```python
from build123d import *

# Parameters (mm, degrees)
CIRPATTERN1_COUNT              = 8
F_1_4_0_2500_DOWEL_HOLE1_D     = 6.35
F_1_4_0_2500_DOWEL_HOLE1_DEPTH = 9.906
F_1_4_0_2500_DOWEL_HOLE1_TIP   = 1.907732465


with BuildPart() as part:
    # Sketch1 → Revolve2 (revolve)
    with BuildSketch(Plane.XY, mode=Mode.PRIVATE) as revolve2_sk:
        with BuildLine():
            Line((71.727523602, 109.927507641), (76.194467874, 109.927507641))
            Line((76.194467874, 109.927507641), (76.194467874, -212.127513222))
            Line((76.194467874, -212.127513222), (53.881527661, -212.127513222))
            Line((53.881527661, -212.127513222), (53.881527661, -59.727513222))
            add(Edge.make_bspline(
                [(53.881527661, -59.727513222), (53.88152643, -59.656983156), (53.880997287, -59.515406102), (53.878621437, -59.181564616), (53.872296838, -58.904795492), (53.862811351, -58.532567487), (53.850168453, -58.212837621), (53.830417626, -57.781594442), (53.800405285, -57.280959899), (53.756193121, -56.687998165), (53.677288452, -55.848480365), (53.577426861, -55.00816586), (53.456675786, -54.17243543), (53.286810822, -53.172425239), (53.092064187, -52.177442821), (52.86637512, -51.188539083), (52.610014224, -50.207489038), (52.32928934, -49.23307774), (52.024348739, -48.265969223), (51.633537831, -47.149135067), (51.139520361, -45.890408405), (50.598733752, -44.650968803), (50.012060927, -43.432701525), (49.38012023, -42.237093238), (48.704125229, -41.066154878), (47.984475519, -39.920972657), (47.223102138, -38.804076239), (46.51986906, -37.851451785), (45.893537937, -37.055672122), (45.35281768, -36.403381282), (44.915126948, -35.894247632), (44.514776189, -35.446992657), (44.181457503, -35.084631185), (43.873924624, -34.760340151), (43.674072406, -34.55154945), (43.444392072, -34.318516287), (43.343783151, -34.217162055), (43.293911001, -34.167289665)],
                knots=[0.082637729, 0.082637729, 0.082637729, 0.082637729, 0.082637729, 0.092574926, 0.102512123, 0.11244932, 0.122386517, 0.132323714, 0.142260911, 0.162135305, 0.182009699, 0.201884093, 0.24163288, 0.261507274, 0.281381668, 0.321130456, 0.360879243, 0.380753637, 0.400628031, 0.440376819, 0.480125606, 0.519874394, 0.559623181, 0.599371969, 0.639120757, 0.678869544, 0.718618332, 0.75836712, 0.798115907, 0.817990301, 0.837864695, 0.857739089, 0.877613483, 0.88755068, 0.897487877, 0.907425074, 0.91736227, 0.91736227, 0.91736227, 0.91736227, 0.91736227], degree=4))
            Line((43.293911001, -34.167289665), (34.686282803, -25.559661468))
            add(Edge.make_bspline(
                [(24.099067874, 0.000160672), (24.099069105, -0.070367974), (24.099598252, -0.213423517), (24.101973937, -0.543022243), (24.108298331, -0.823999723), (24.117783452, -1.194661398), (24.130425744, -1.513274385), (24.146225968, -1.86177893), (24.165181227, -2.193546199), (24.192818841, -2.617908727), (24.232287047, -3.121873274), (24.303299707, -3.879818002), (24.423126678, -4.886289716), (24.599486044, -6.056550088), (24.850885233, -7.385005743), (25.151795313, -8.703413844), (25.501770623, -10.009476539), (25.900360983, -11.301658928), (26.346945392, -12.577938667), (26.841003323, -13.836726817), (27.381673122, -15.076036463), (27.968479387, -16.294449129), (28.600139398, -17.489778131), (29.276532396, -18.661127096), (29.995445102, -19.805582737), (30.758021999, -20.923699417), (31.459167193, -21.874251104), (32.088736123, -22.673284825), (32.624128416, -23.320261484), (33.072255768, -23.839844364), (33.508450026, -24.329655594), (33.935826121, -24.788323739), (34.24555864, -25.11370766), (34.536859958, -25.409488397), (34.636412426, -25.509789283), (34.686282803, -25.559661468)],
                knots=[0.082637729, 0.082637729, 0.082637729, 0.082637729, 0.082637729, 0.092574926, 0.102512123, 0.11244932, 0.122386517, 0.132323714, 0.142260911, 0.152198108, 0.162135305, 0.182009699, 0.201884093, 0.24163288, 0.281381668, 0.321130456, 0.360879243, 0.400628031, 0.440376819, 0.480125606, 0.519874394, 0.559623181, 0.599371969, 0.639120757, 0.678869544, 0.718618332, 0.75836712, 0.798115907, 0.817990301, 0.837864695, 0.857739089, 0.877613483, 0.897487877, 0.907425074, 0.91736227, 0.91736227, 0.91736227, 0.91736227, 0.91736227], degree=4))
            add(Edge.make_bspline(
                [(24.099067874, 0.000160672), (24.0990685, 0.036053324), (24.099606331, 0.110274362), (24.102023723, 0.267801742), (24.108461568, 0.427224789), (24.120533599, 0.646924939), (24.141435087, 0.901594), (24.175184719, 1.202697945), (24.226499305, 1.54221117), (24.290543701, 1.881157449), (24.367141601, 2.216515092), (24.456323571, 2.549400093), (24.557741413, 2.878253317), (24.671619071, 3.203507713), (24.797196771, 3.523787829), (24.935285977, 3.839827405), (25.084070301, 4.149442857), (25.246012222, 4.454943795), (25.416488505, 4.751462248), (25.602514721, 5.045864533), (25.79178827, 5.325679608), (26.004405474, 5.610888215), (26.178876374, 5.83307432), (26.366345756, 6.050112309), (26.504555248, 6.208802318), (26.67044207, 6.382282451), (26.744520261, 6.458639514), (26.795279203, 6.509400323)],
                knots=[0.082568816, 0.082568816, 0.082568816, 0.082568816, 0.082568816, 0.102426634, 0.122284453, 0.142142271, 0.162000089, 0.201715725, 0.241431362, 0.281146998, 0.320862634, 0.360578271, 0.400293907, 0.440009544, 0.47972518, 0.519440816, 0.559156453, 0.598872089, 0.638587725, 0.678303362, 0.718018998, 0.757734635, 0.797450271, 0.837165907, 0.857023726, 0.876881544, 0.91659718, 0.91659718, 0.91659718, 0.91659718, 0.91659718], degree=4))
            add(Edge.make_bspline(
                [(26.795279203, 6.509400323), (49.261401403, 34.636114842), (71.727523602, 109.927507641)],
                knots=[0, 0, 0, 1, 1, 1], degree=2))
        make_face()
    revolve(revolve2_sk.sketch.rotate(Axis((-0.005532126, 165.815985114, 0), (0, -1, 0)), 180), axis=Axis((-0.005532126, 165.815985114, 0), (0, -1, 0)))

    # Sketch4 → 3/8-24 Tapped Hole1 (revolve, cut)
    with BuildSketch(Plane(origin=(65.2, -212.127513222, 0), x_dir=(0, 0, -1), z_dir=(1, 0, 0))):
        Polygon((0, 0), (0, 27.533468714), (4.2164, 25), (4.2164, 0), align=None)
    f_3_8_24_tapped_hole1 = revolve(axis=Axis((65.2, -218.477513222, 0), (0, 1, 0)), mode=Mode.SUBTRACT)

    # CirPattern1: 3/8-24 Tapped Hole1 ×8 about axis
    cirpattern1_axis = Axis((0, -228.487022387, 0), (-1.634718801334702e-05, 0.9999999998663848, 0))
    for i in range(1, CIRPATTERN1_COUNT):
        add(f_3_8_24_tapped_hole1.rotate(cirpattern1_axis, i * 360 / CIRPATTERN1_COUNT), mode=Mode.SUBTRACT)

    # 1/4 (0.2500) Dowel Hole1
    with Locations(Plane(origin=(0, -212.127513222, 0), x_dir=(-1, 0, 0), z_dir=(0, -1, 0))):
        with Locations((-60.236831784, 24.951234372), (60.23705925, -24.95068522)):
            Hole(F_1_4_0_2500_DOWEL_HOLE1_D / 2, depth=F_1_4_0_2500_DOWEL_HOLE1_DEPTH)
            with Locations((0, 0, -(F_1_4_0_2500_DOWEL_HOLE1_DEPTH + F_1_4_0_2500_DOWEL_HOLE1_TIP / 2))):  # 118° drill point
                Cone(0, F_1_4_0_2500_DOWEL_HOLE1_D / 2, F_1_4_0_2500_DOWEL_HOLE1_TIP, mode=Mode.SUBTRACT)


solid = part.part
```
Can you work these out from the model? Positions are in its coordinate system, mm. Coordinates: 2 decimals unless noted, no trailing zeros. Write each loop counter-clockwise with the first axis right and the second up, starting at its lowest first coordinate (ties: lowest second). Pieces come first, ordered by that corner, then holes. Notation, with made-up numbers: (83, 18) - (124, 18) arc R15 ccw to (124, 32) - close; hole circle Ø6 at (-3, -20). An arc over 180 degrees is marked (long way). Return JSON: item names as keys, results as strings.
Q1. I'm going to push flat-ended pins straight in: pin 1 Ø11 at (x, z) = (-65.2, 0) entering from -Y; pin 2 Ø6 at (y, z) = (45.5, -59) entering from +X; pin 3 Ø5 at (x, z) = (-19, 21) entering from -Y; pin 4 Ø3 at (x, z) = (38.5, -4.5) entering from +Y. Where does each tip first touch, or does it pass through?
Computed values:
{"pin 1": "stops at y = -212.13", "pin 2": "stops at x = 51.67", "pin 3": "stops at y = -20.98", "pin 4": "stops at y = 27.61"}
Q2. If we section it at A-A (y = -94.5): Please give me the cut outline in (x, z), then the cut area to 3 significant figures.
Computed values:
{"outline": "circle Ø152.4 at (-0.01, 0); hole circle Ø107.77 at (-0.01, 0)", "area": "9,120 mm2"}
Q3. Thinking about a two-plate mould opening in Z: for faces 1 (the conical face through (-65.92, -185.04, -0.16)), 2 (the cylindrical face through (16.51, -53.35, 74.39)), which applies, +Z half, -Z half, draft (parallel to the pull), parting line (faces both ways), or undercut?
Computed values:
{"face 1": "undercut", "face 2": "parting line"}
Q4. Please list where these lines run through material, in increasing order: L1, parallel to X at y = -185, z = 1; L2, parallel to Z at x = 22, y = 89; L3, parallel to Z at x = -1.5, y = -97.5. Write a range as from..to.
Computed values:
{"L1": "x = -76.2..-53.88, 53.87..76.19", "L2": "z = -72.95..-61.36, 61.36..72.95", "L3": "z = -76.19..-53.87, 53.87..76.19"}
